For this review, take the finished solid that the model builds, in its own axes (mm). A direction names the side the tool comes from. Coordinates: 2 decimals unless noted, no trailing zeros. Write each loop counter-clockwise with the first axis right and the second up, starting at its lowest first coordinate (ties: lowest second). Pieces come first, ordered by that corner, then holes.
```python
from build123d import *

# Parameters (mm, degrees)
F0_W      = 152.4
F0_H      = 152.4
F1_DEPTH  = 2.6416
F2_W      = 2.6416
F2_H      = 44.45
F3_DEPTH  = 76.2
F4_R      = 57.785
F5_DEPTH  = 25.4
F6_R      = 50.8
F7_R      = 4.953
F8_DEPTH  = 25.4
F10_DEPTH = 2.6416
F11_R     = 12.7


with BuildPart() as f1:
    # F0 (on Front) → F1 (new body)
    with BuildSketch(Plane.XZ):
        Rectangle(F0_W, F0_H)
    extrude(amount=F1_DEPTH)

    # F2 (on face) → F3 (join)
    with BuildSketch(Plane(origin=(0, 0, 0), x_dir=(-1, 0, 0), z_dir=(0, 1, 0))):
        with Locations((-74.8792, -53.975)):
            Rectangle(F2_W, F2_H)
    extrude(amount=F3_DEPTH)

    # F4 (on face) → F5 (cut)
    with BuildSketch(Plane.XZ.offset(2.6416)):
        Circle(F4_R)
    extrude(amount=-F5_DEPTH, mode=Mode.SUBTRACT)

    # F6
    f6_edges = [f1.edges().sort_by_distance(p)[0] for p in [
        (76.2, -1.3208, 76.2),
        (-76.2, -1.3208, 76.2),
        (-76.2, -1.3208, -76.2),
    ]]
    fillet(f6_edges, radius=F6_R)

    # F7 (on face) → F8 (cut)
    with BuildSketch(Plane(origin=(73.5584, 0, 0), x_dir=(0, -1, 0), z_dir=(-1, 0, 0))):
        with Locations((-11.6586, -55.5625)):
            Circle(F7_R)
        with Locations((-62.4586, -55.5625)):
            Circle(F7_R)
    extrude(amount=-F8_DEPTH, mode=Mode.SUBTRACT)

    # F9 (on face) → F10 (join)
    with BuildSketch(Plane.YZ.offset(76.2)):
        Polygon((18.402247, 25.4), (0, 25.4), (0, -31.75), (76.2, -31.75), align=None)
    extrude(amount=-F10_DEPTH)

    # F11
    f11_edges = [f1.edges().sort_by_distance(p)[0] for p in [
        (74.8792, 76.2, -76.2),
        (74.8792, 76.2, -31.75),
        (74.8792, 18.402247, 25.4),
    ]]
    fillet(f11_edges, radius=F11_R)


solid = f1.part
```
1) Consider section A-A (x = 0). Give the boundary of the cut face in (y, z) (3 decimals), then the cut area to 3 significant figures.
2) Consider section B-B (z = -17.5). Give the boundary of the cut face in (x, y).
3) Consider section D-D (z = 0). Give the boundary of the cut face in (x, y) (3 decimals).
4) Clearance check with flat-ended pins moving along their axes: P1, Ø10, axis at x = -61, z = 47, coming from the +Y side; P2, Ø3, axis at x = 75, y = 5.5, coming from the +Z side; P3, Ø8, axis at y = 62.46, z = -55.56, coming from the +X side; P4, Ø13, axis at y = 11.66, z = -55.56, coming from the -X side. State where each tip first meets the part, or that it passes through.
5) Consider section C-C (y = 11). Give the boundary of the cut face in (x, z).
6) Tool access review of faces 1 (the face through (73.558, 29, -36)), 2 (the face through (61.714, -1.339, 60.924)): name each direction out of +Z, -Z, +X, -X, +Y, -Y from which nothing blocks a thin tool from reaching the whole face with its end or side.
7) The part is to be moulded in two halves that separate along X. For faces 3 (the face through (74.9, 47.62, -3.49)), 4 (the face through (-60.924, -1.339, -61.714)), 5 (the face through (-12.53, -1.34, -56.41)), say which applies: pulls with the +X half, pulls with the -X half, needs draft (parallel to the pull), parting line crosses it, or undercut.
8) For L1, parallel to Z at x = 0, y = -1.9 (3 decimals); L2, parallel to X at y = 23, z = -22.5; L3, parallel to Y at x = 52.5, z = -40, list the stretches that pass through material, from the lowest coordinate up.
Results:
1. outline: (-2.642, -76.2) - (0, -76.2) - (0, -57.785) - (-2.642, -57.785) - close; (-2.642, 57.785) - (0, 57.785) - (0, 76.2) - (-2.642, 76.2) - close
1. area: 97.3 mm2
2. outline: (-76.2, -2.64) - (-55.07, -2.64) - (-55.07, 0) - (-76.2, 0) - close; (55.07, -2.64) - (76.2, -2.64) - (76.2, 61.79) - (73.56, 61.79) - (73.56, 0) - (55.07, 0) - close
3. outline: (-76.2, -2.642) - (-57.785, -2.642) - (-57.785, 0) - (-76.2, 0) - close; (57.785, -2.642) - (76.2, -2.642) - (76.2, 44.09) - (73.558, 44.09) - (73.558, 0) - (57.785, 0) - close
4. P1: stops at y = 0
4. P2: stops at z = 25.4
4. P3: passes through
4. P4: stops at x = 73.56
5. outline: (73.56, -76.2) - (76.2, -76.2) - (76.2, -60.47) - (73.56, -60.47) - close; (73.56, -50.65) - (76.2, -50.65) - (76.2, 25.4) - (73.56, 25.4) - close
6. face 1: +Z, -Z, -X, +Y
6. face 2: +Z, +X, +Y, -Y
7. face 3: needs draft
7. face 4: pulls with the -X half
7. face 5: undercut
8. L1: z = -76.2 to -57.785, 57.785 to 76.2
8. L2: x = 73.56 to 76.2
8. L3: y = -2.64 to 0
